Job drawing, mm, ordinate dimensions from the low corner. One solid piece. Give positions to 0.01 mm unless a question says otherwise; leave off trailing zeros. Loops run counter-clockwise (first coordinate to the right, second up) from the corner with the lowest first, then second, coordinate; pieces in that order, holes last. Notation, with made-up numbers: M 14,64 L 27,64 A19 cw 27,101 Z; hole C 59,49.25 d9. An arc over 180 degrees is marked long. Put each result on its own line as item: value.
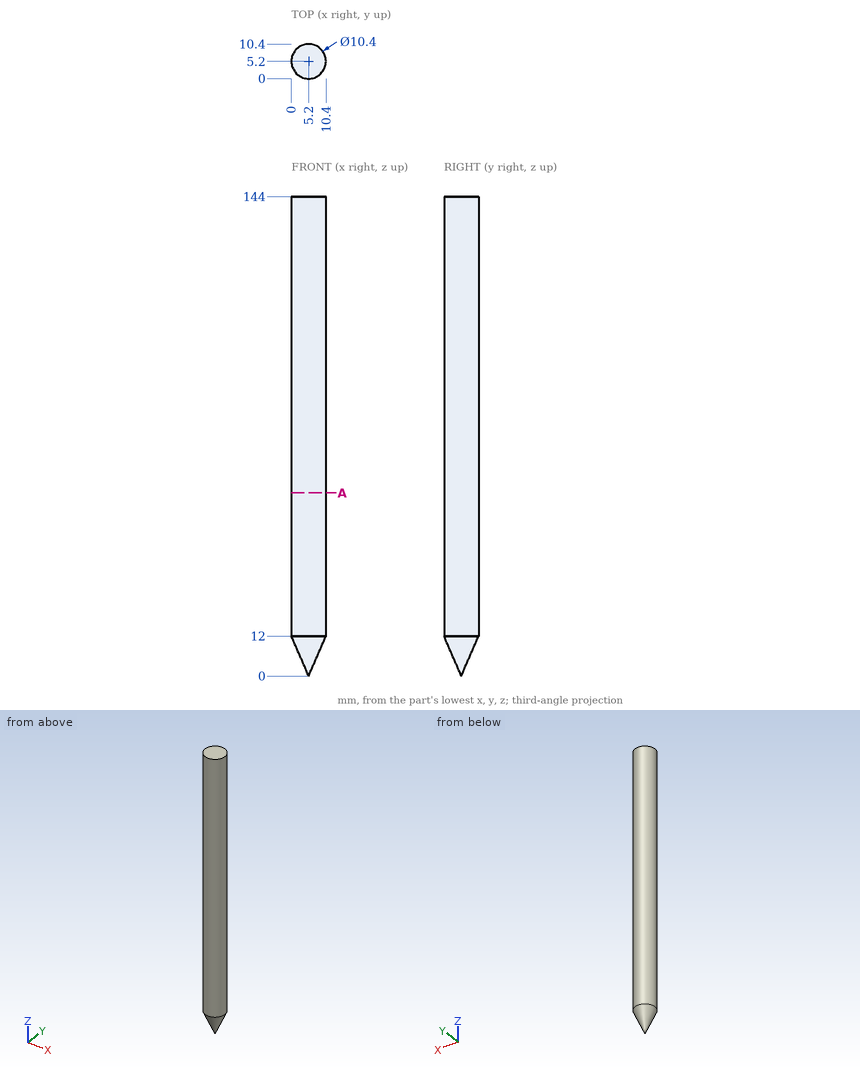
Q1. Drop a flat-ended pin along its axis: pin 1 Ø1 at (x, y) = (4.5, 3) entering from -Z. Give the stop position or say it passes through.
Here are the results:
pin 1: z = 4.17
Q2. Probe line 1 (Y direction, x = 4.75, z = 99.5); line 2 (X direction, y = 4, z = 71.5). List the from-to ranges inside material, lowest first. Write a range as from..to.
Here are the results:
line 1: 0.02..10.38
line 2: 0.14..10.26
Q3. Slice it at A-A (z = 55). List the corners of the cut face in (x, y), and give its area (3 significant figures).
Here are the results:
outline: C 5.2,5.2 d10.4
area: 84.9 mm²
